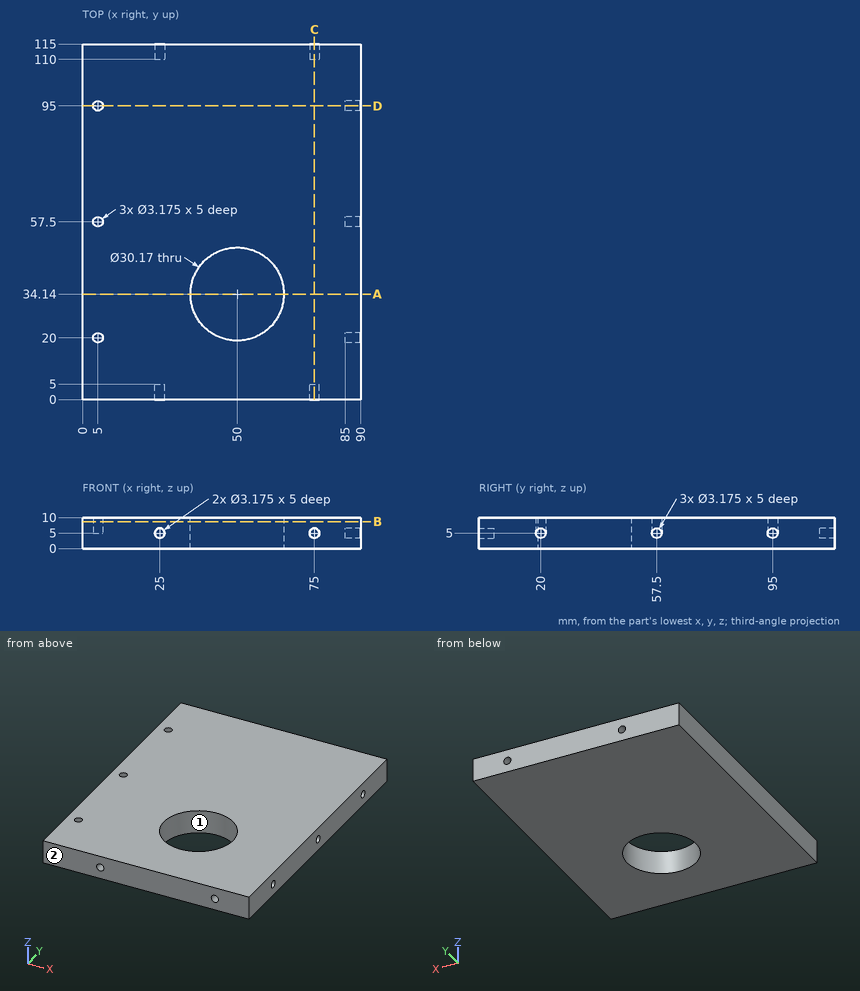
Job drawing, mm, ordinate dimensions from the low corner. One solid piece. Round coordinates to 2 decimals unless told otherwise and drop trailing zeros. Order: outer loops, then holes, each group sorted by start corner. A loop starts at its lowest first (then second) coordinate and runs counter-clockwise, first axis right, second up. Notation, with made-up numbers: (32.5, 42) -> (88.5, 42) arc R34 ccw to (88.5, 72) -> close; hole circle Ø7 at (-23.75, 85.25). An arc over 180 degrees is marked (long way). Answer in a Markdown table with one row per item.
1) Wall check: L1, parallel to X at y = 113.5, z = 5; L2, parallel to Y at x = 5, z = 6.8; L3, parallel to Z at x = 75, y = 111.45. Give the ranges that are in metal, low to high.
Values:
| item | result |
|---|---|
| L1 | 0 to 23.41, 26.59 to 73.41, 76.59 to 90 |
| L2 | 0 to 18.41, 21.59 to 55.91, 59.09 to 93.41, 96.59 to 115 |
| L3 | 0 to 3.41, 6.59 to 10 |
2) Band-saw the part on B-B on z = 8.75. Give the cut face in (x, y) (1 decimal), and give its area (3 significant figures).
Values:
| item | result |
|---|---|
| outline | (0, 0) -> (90, 0) -> (90, 115) -> (0, 115) -> close; hole circle Ø3.2 at (5, 20); hole circle Ø3.2 at (5, 57.5); hole circle Ø3.2 at (5, 95); hole circle Ø30.2 at (50, 34.1) |
| area | 9,610 mm2 |
3) Band-saw the part on C-C on x = 75. Give the cut face in (y, z), and give its area (3 significant figures).
Values:
| item | result |
|---|---|
| outline | (0, 0) -> (115, 0) -> (115, 3.41) -> (110, 3.41) -> (110, 6.59) -> (115, 6.59) -> (115, 10) -> (0, 10) -> (0, 6.59) -> (5, 6.59) -> (5, 3.41) -> (0, 3.41) -> close |
| area | 1,120 mm2 |
4) Band-saw the part on A-A on y = 34.14. Give the cut face in (x, z) (3 decimals), and give its area (3 significant figures).
Values:
| item | result |
|---|---|
| outline | (0, 0) -> (34.915, 0) -> (34.915, 10) -> (0, 10) -> close; (65.085, 0) -> (90, 0) -> (90, 10) -> (65.085, 10) -> close |
| area | 598 mm2 |
5) Pin check, flat tips, straight feed: P1, Ø1.6, axis at x = 5, y = 58, coming from the +Z side; P2, Ø1.9, axis at x = 75, z = 5, coming from the -Y side; P3, Ø2.5, axis at y = 20, z = 5, coming from the +X side. Stop position of each tip, or through.
Values:
| item | result |
|---|---|
| P1 | z = 5 |
| P2 | y = 5 |
| P3 | x = 85 |
6) Band-saw the part on D-D on y = 95. Give the cut face in (x, z), and give its area (3 significant figures).
Values:
| item | result |
|---|---|
| outline | (0, 0) -> (90, 0) -> (90, 3.41) -> (85, 3.41) -> (85, 6.59) -> (90, 6.59) -> (90, 10) -> (6.59, 10) -> (6.59, 5) -> (3.41, 5) -> (3.41, 10) -> (0, 10) -> close |
| area | 868 mm2 |
7) Mould opens along X. For the marked faces 1 and 2 say: released by +X, released by -X, zero draft, split by the parting line, or undercut.
Values:
| item | result |
|---|---|
| face 1 | undercut |
| face 2 | zero draft |
